The listing builds one solid part. Answer for the finished solid, in the listing's coordinates (mm). A direction names the side the tool comes from. Give positions to 0.01 mm unless a question says otherwise; leave off trailing zeros. Order: outer loops, then holes, each group sorted by start corner. A loop starts at its lowest first (then second) coordinate and runs counter-clockwise, first axis right, second up. Notation, with made-up numbers: (40, 38.25) - (64, 38.25) arc R14 ccw to (64, 43.25) - close; hole circle Ø8 at (-30, 12.25). An arc over 180 degrees is marked (long way). Use CSV: the item, a comma, the result in double quotes.
```python
from build123d import *

# Parameters (mm, degrees)
SKETCH2_W           = 49.75
SKETCH2_H           = 40
BOSS_EXTRUDE1_DEPTH = 3
SKETCH2_4_W         = 3
SKETCH2_4_H         = 40
BOSS_EXTRUDE3_DEPTH = 11.9
SKETCH2_5_W         = 3
SKETCH2_5_H         = 40
BOSS_EXTRUDE4_DEPTH = 13
CUT_EXTRUDE1_REACH  = 57.173
SKETCH3_R           = 1.1
SKETCH3_W           = 24.5
SKETCH3_H           = 6.4
SKETCH4_R           = 1.6
CUT_EXTRUDE2_DEPTH  = 3


with BuildPart() as part:
    # Sketch2 → Boss-Extrude1 (new body)
    with BuildSketch(Plane(origin=(0, 0, 0), x_dir=(1, 0, 0), z_dir=(0, 1, 0))):
        Rectangle(SKETCH2_W, SKETCH2_H)
    extrude(amount=BOSS_EXTRUDE1_DEPTH)

    # Sketch2<4> → Boss-Extrude3 (add)
    with BuildSketch(Plane(origin=(0, 0, 0), x_dir=(1, 0, 0), z_dir=(0, 1, 0))):
        with Locations((9.625, 0)):
            Rectangle(SKETCH2_4_W, SKETCH2_4_H)
        with Locations((-23.375, 0)):
            Rectangle(SKETCH2_4_W, SKETCH2_4_H)
    extrude(amount=-BOSS_EXTRUDE3_DEPTH)

    # Sketch2<5> → Boss-Extrude4 (add)
    with BuildSketch(Plane(origin=(0, 0, 0), x_dir=(1, 0, 0), z_dir=(0, 1, 0))):
        with Locations((23.375, 0)):
            Rectangle(SKETCH2_5_W, SKETCH2_5_H)
    extrude(amount=BOSS_EXTRUDE4_DEPTH)

    # Cut-Extrude1: up to this face of the body (flat: up to its plane)
    cut_extrude1_end = Plane(part.part.faces().sort_by_distance((11.125, -5.95, 0))[0])
    # Sketch3 → Cut-Extrude1 (cut, up to the picked face)
    with BuildSketch(Plane.ZY.offset(24.875), mode=Mode.PRIVATE) as cut_extrude1_sk1:
        with Locations((-8.5, -2.8)):
            Circle(SKETCH3_R)
    cut_extrude1_tool1 = split(extrude(cut_extrude1_sk1.sketch, amount=-CUT_EXTRUDE1_REACH, mode=Mode.PRIVATE), bisect_by=cut_extrude1_end, keep=Keep.BOTH, mode=Mode.PRIVATE)
    # Sketch3 → Cut-Extrude1 (cut, up to the picked face)
    with BuildSketch(Plane.ZY.offset(24.875), mode=Mode.PRIVATE) as cut_extrude1_sk2:
        with Locations((-15, -9.1)):
            Circle(SKETCH3_R)
    cut_extrude1_tool2 = split(extrude(cut_extrude1_sk2.sketch, amount=-CUT_EXTRUDE1_REACH, mode=Mode.PRIVATE), bisect_by=cut_extrude1_end, keep=Keep.BOTH, mode=Mode.PRIVATE)
    # Sketch3 → Cut-Extrude1 (cut, up to the picked face)
    with BuildSketch(Plane.ZY.offset(24.875), mode=Mode.PRIVATE) as cut_extrude1_sk3:
        with Locations((0, -8.7)):
            Rectangle(SKETCH3_W, SKETCH3_H)
    cut_extrude1_tool3 = split(extrude(cut_extrude1_sk3.sketch, amount=-CUT_EXTRUDE1_REACH, mode=Mode.PRIVATE), bisect_by=cut_extrude1_end, keep=Keep.BOTH, mode=Mode.PRIVATE)
    cut_extrude1_1 = cut_extrude1_tool1.solids().sort_by(Axis((-24.875, -2.8, -8.5), (1, 0, 0)))[0]
    add(cut_extrude1_1, mode=Mode.SUBTRACT)
    cut_extrude1_2 = cut_extrude1_tool2.solids().sort_by(Axis((-24.875, -9.1, -15), (1, 0, 0)))[0]
    add(cut_extrude1_2, mode=Mode.SUBTRACT)
    cut_extrude1_3 = cut_extrude1_tool3.solids().sort_by(Axis((-24.875, -8.7, 0), (1, 0, 0)))[0]
    add(cut_extrude1_3, mode=Mode.SUBTRACT)
    cut_extrude1 = cut_extrude1_1 + cut_extrude1_2 + cut_extrude1_3  # Cut-Extrude1 as one shape, for the pattern or mirror that repeats it

    # Sketch4 → Cut-Extrude2 (cut)
    with BuildSketch(Plane.ZY.offset(-21.875)):
        with Locations((-14.75, 8)):
            Circle(SKETCH4_R)
    cut_extrude2 = extrude(amount=-CUT_EXTRUDE2_DEPTH, mode=Mode.SUBTRACT)

    # Mirror2: Cut-Extrude1, Cut-Extrude2 across plane
    add(cut_extrude1.mirror(Plane.XY), mode=Mode.SUBTRACT)
    add(cut_extrude2.mirror(Plane.XY), mode=Mode.SUBTRACT)


solid = part.part
```
Item 1: Each of these flat-tipped pins is pushed along its axis until it touches: pin 1 (1.9 mm diameter, centred on y = 8, z = 14.75, fed in from -X); pin 2 (13 mm diameter, centred on y = -7, z = -3.5, fed in from +X) (3 decimals); pin 3 (13 mm diameter, centred on y = -6, z = -9, fed in from -X) (3 decimals); pin 4 (5 mm diameter, centred on x = -7, z = 6, fed in from +Y). Where does it stop, or does it pass through?
Taken from the geometry:
pin 1,"through"
pin 2,"x = 11.125"
pin 3,"x = -24.875"
pin 4,"y = 3"
Item 2: The part is cut by section A-A (y = -2.8). Give the vertices of the cut face in (x, z) (3 decimals).
Taken from the geometry:
outline,"(-24.875, -20) - (-21.875, -20) - (-21.875, -9.6) - (-24.875, -9.6) - close; (-24.875, -7.4) - (-21.875, -7.4) - (-21.875, 7.4) - (-24.875, 7.4) - close; (-24.875, 9.6) - (-21.875, 9.6) - (-21.875, 20) - (-24.875, 20) - close; (8.125, -20) - (11.125, -20) - (11.125, -9.6) - (8.125, -9.6) - close; (8.125, -7.4) - (11.125, -7.4) - (11.125, 7.4) - (8.125, 7.4) - close; (8.125, 9.6) - (11.125, 9.6) - (11.125, 20) - (8.125, 20) - close"
Item 3: Which of the six approach directions +Z, -Z, +X, -X, +Y, -Y give full straight-line access (tool end or side, diameter ignored) to faces 5 (the face through (18, 0, 0)), 6 (the face through (-23.396, -3.221, 7.484)), 7 (the face through (-23, -5.5, 0))?
Taken from the geometry:
face 5,"+Z, -Z, +X, -Y"
face 6,"+X, -X"
face 7,"+X, -X, -Y"
Item 4: The part is cut by section B-B (z = -8.5). Give the vertices of the cut face in (x, y) (3 decimals), and give its area (3 significant figures).
Taken from the geometry:
outline,"(-24.875, -5.5) - (-21.875, -5.5) - (-21.875, -3.9) - (-24.875, -3.9) - close; (-24.875, -1.7) - (-21.875, -1.7) - (-21.875, 0) - (8.125, 0) - (8.125, -1.7) - (11.125, -1.7) - (11.125, 0) - (24.875, 0) - (24.875, 13) - (21.875, 13) - (21.875, 3) - (-24.875, 3) - close; (8.125, -5.5) - (11.125, -5.5) - (11.125, -3.9) - (8.125, -3.9) - close"
area,"199 mm^2"
Item 5: The part is cut by section D-D (z = 1.5). Give the vertices of the cut face in (x, y) (3 decimals), and give its area (3 significant figures).
Taken from the geometry:
outline,"(-24.875, -5.5) - (-21.875, -5.5) - (-21.875, 0) - (8.125, 0) - (8.125, -5.5) - (11.125, -5.5) - (11.125, 0) - (24.875, 0) - (24.875, 13) - (21.875, 13) - (21.875, 3) - (-24.875, 3) - close"
area,"212 mm^2"
Item 6: Find the intervals of material crossed by line 1 along Y through (x, z) = (8.8, 8.5); line 2 along Y through (x, z) = (9, 15); line 3 along X through (y, z) = (-0.75, 9) (3 decimals), in increasing order.
Taken from the geometry:
line 1,"-5.5 to -3.9, -1.7 to 3"
line 2,"-11.9 to -10.2, -8 to 3"
line 3,"-24.875 to -21.875, 8.125 to 11.125"
Item 7: The part is cut by section C-C (y = -9.1). Count the separate pieces of the cut face and the enclosed holes in it, and give its area (3 significant figures).
Taken from the geometry:
separate pieces,"8"
enclosed holes,"0"
area,"66.6 mm^2"
Item 8: The mould has two halves that part along X. Classify faces 1 (the face through (21.875, 8, 0)), 2 (the face through (8.125, -5, 0)), 3 (the face through (-21.875, -5, 0)), 4 (the face through (-23, -11.9, -16)): +X half, -X half, draft (parallel to the pull), parting line (faces both ways), or undercut.
Taken from the geometry:
face 1,"-X half"
face 2,"undercut"
face 3,"undercut"
face 4,"draft"
